Source: three-view drawing plus pictorial views. Frame: mm from the lowest corner of the part. A direction names the side the tool comes from. Give positions to 0.01 mm unless a question says otherwise; leave off trailing zeros. Loops run counter-clockwise (first coordinate to the right, second up) from the corner with the lowest first, then second, coordinate; pieces in that order, holes last. Notation, with made-up numbers: (7, 45) - (34, 45) arc R30 cw to (34, 72) - close; hole circle Ø9 at (43, 66). An arc over 180 degrees is marked (long way). Answer in a Markdown table with one row per item.
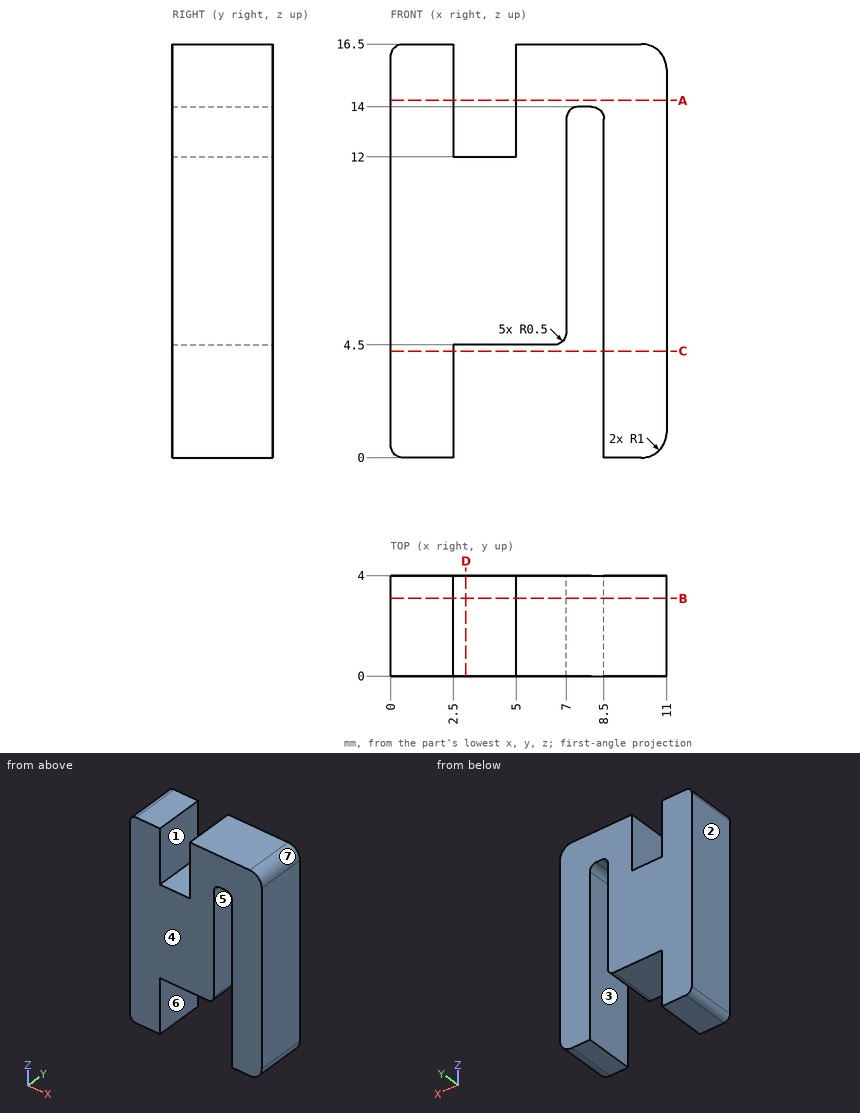
Q1. First-contact query: pin 1 (1.2 mm diameter, centred on y = 2.5, z = 13.5, fed in from -X); pin 2 (0.8 mm diameter, centred on x = 3.5, y = 2.5, fed in from +Z). Flat tips, straight axial feed; report the tip coordinate or a pass-through.
Check values:
| item | result |
|---|---|
| pin 1 | x = 0 |
| pin 2 | z = 12 |
Q2. Material intervals for line 1 along X through (y, z) = (2.2, 13.5); line 2 along X through (y, z) = (2.2, 6.75); line 3 along X through (y, z) = (3.1, 15.5), sorted ascending.
Check values:
| item | result |
|---|---|
| line 1 | 0 to 2.5, 5 to 7, 8.5 to 11 |
| line 2 | 0 to 7, 8.5 to 11 |
| line 3 | 0 to 2.5, 5 to 11 |
Q3. Cut plane A-A (z = 14.25). Output: boundary loops of the cut face in (x, y).
Check values:
| item | result |
|---|---|
| outline | (0, 0) - (2.5, 0) - (2.5, 4) - (0, 4) - close; (5, 0) - (11, 0) - (11, 4) - (5, 4) - close |
Q4. Reachability of the marked faces 1, 2 and 3 from +Z, -Z, +X, -X, +Y, -Y: full face, straight path, thin tool, end or side. Return the list, or none.
Check values:
| item | result |
|---|---|
| face 1 | +Z, +Y, -Y |
| face 2 | +Z, -Z, -X, +Y, -Y |
| face 3 | -Z, +Y, -Y |
Q5. Cut plane D-D (x = 3). Output: boundary loops of the cut face in (y, z).
Check values:
| item | result |
|---|---|
| outline | (0, 4.5) - (4, 4.5) - (4, 12) - (0, 12) - close |
Q6. Cut plane B-B (y = 3.1). Output: boundary loops of the cut face in (x, z), and give its area (3 significant figures).
Check values:
| item | result |
|---|---|
| outline | (0, 0.5) arc R0.5 ccw to (0.5, 0) - (2.5, 0) - (2.5, 4.5) - (6.5, 4.5) arc R0.5 ccw to (7, 5) - (7, 13.5) arc R0.5 cw to (7.5, 14) - (8, 14) arc R0.5 cw to (8.5, 13.5) - (8.5, 0) - (10, 0) arc R1 ccw to (11, 1) - (11, 15.5) arc R1 ccw to (10, 16.5) - (5, 16.5) - (5, 12) - (2.5, 12) - (2.5, 16.5) - (0.5, 16.5) arc R0.5 ccw to (0, 16) - close |
| area | 129 mm² |
Q7. Draft query along X for the marked faces 4, 5, 6 and 7. Return one class per face: pulls with the +X half, pulls with the -X half, needs draft (parallel to the pull), parting line crosses it, or undercut.
Check values:
| item | result |
|---|---|
| face 4 | needs draft |
| face 5 | undercut |
| face 6 | undercut |
| face 7 | pulls with the +X half |
Q8. Cut plane C-C (z = 4.25). Output: boundary loops of the cut face in (x, y).
Check values:
| item | result |
|---|---|
| outline | (0, 0) - (2.5, 0) - (2.5, 4) - (0, 4) - close; (8.5, 0) - (11, 0) - (11, 4) - (8.5, 4) - close |
